Part model, mm, in its own coordinate system. Coordinates: 2 decimals unless noted, no trailing zeros. Loops run counter-clockwise (first coordinate to the right, second up) from the corner with the lowest first, then second, coordinate; pieces in that order, holes last. Notation, with made-up numbers: (-32, 83.25) -> (-27, 83.25) arc R34 ccw to (-27, 120.25) -> close; hole circle Ø3 at (-27, -36.75). An arc over 180 degrees is marked (long way). One line per item, written item: value. Start each with the question number.
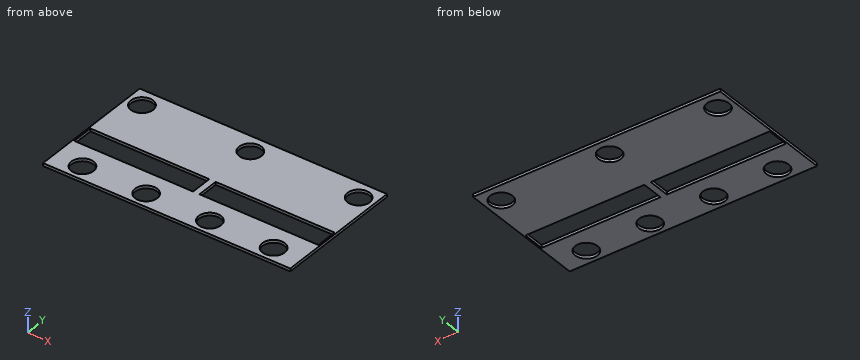
from build123d import *

# Parameters (mm, degrees)
SKETCH14_W                        = 80
SKETCH14_H                        = 42
SKETCH14_W_2                      = 3.75
SKETCH14_H_2                      = 3.75
BASE_WITH_CUTOUTS_DEPTH           = 3
SKETCH15_W                        = 4.3
SKETCH15_H                        = 4.8
SIPM_CUTOUTS_DEPTH                = 48.265209192
PADDLE_SUPPORT_TAPERS_DEPTH       = 2
SKETCH17_W                        = 80
SKETCH17_H                        = 25
PADDLE_SUPPORT_TOP_DEPTH          = 1
PADDLE_START                      = -4
SKETCH17_2_W                      = 80
SKETCH17_2_H                      = 25
PADDLE_SUPPORT_BOTTOM_DEPTH       = 1
PADDLE_SUPPORT_TAPER_TOP_SIZE     = 0.8
PADDLE_SUPPORT_TAPER_TOP_SIZE2    = 2.4
PADDLE_SUPPORT_TAPER_BOTTOM_SIZE  = 2.4
PADDLE_SUPPORT_TAPER_BOTTOM_SIZE2 = 0.8
SKETCH18_W                        = 4
SKETCH18_H                        = 22
SKETCH18_H_2                      = 14
BASE_THICKNESS_EXPANSION_DEPTH    = 80
BAFFLE_BASE_DEPTH                 = 2
BAFFLE_LIP_DEPTH                  = 2
BAFFLE_CHAMFER_1_2_SIZE           = 1.2
BAFFLE_CHAMFER_0_4_SIZE           = 0.4
INSERT_HOLES_PCB_D                = 3.3
INSERT_HOLES_PCB_DEPTH            = 4.2
INSERT_HOLES_PCB_CBORE_D          = 7
INSERT_HOLES_PCB_CBORE_DEPTH      = 1.4
JOINT_MOD_REACH                   = 56.854
SKETCH29_W                        = 37.3
SKETCH29_H                        = 6.8
CUT_EXTRUDE1_DEPTH                = 1.45
CHAMFER1_SIZE                     = 2
CHAMFER1_SIZE2                    = 5.494954839
SKETCH34_W                        = 81.499638764
SKETCH34_H                        = 0.25
CUT_EXTRUDE2_DEPTH                = 24
M1_6_CLEARANCE_HOLE1_D            = 1.8
SKETCH38_W                        = 104.100396554
SKETCH38_H                        = 54.802140704
CUT_EXTRUDE3_DEPTH                = 55.128573785
CUT_EXTRUDE4_DEPTH                = 0.05
SKETCH40_W                        = 1.2
SKETCH40_H                        = 9
CUT_EXTRUDE5_DEPTH                = 48.190677045
SKETCH41_W                        = 77.6
SKETCH41_H                        = 40.8
CUT_EXTRUDE6_DEPTH                = 0.5


with BuildPart() as part:
    # Sketch14 → BASE WITH CUTOUTS (new body)
    with BuildSketch(Plane.XY):
        with Locations((0, 4)):
            Rectangle(SKETCH14_W, SKETCH14_H)
        with Locations((10.45, 0)):
            Rectangle(SKETCH14_W_2, SKETCH14_H_2, mode=Mode.SUBTRACT)
        with Locations((4.15, 0)):
            Rectangle(SKETCH14_W_2, SKETCH14_H_2, mode=Mode.SUBTRACT)
        with Locations((16.75, 0)):
            Rectangle(SKETCH14_W_2, SKETCH14_H_2, mode=Mode.SUBTRACT)
        with Locations((23.05, 0)):
            Rectangle(SKETCH14_W_2, SKETCH14_H_2, mode=Mode.SUBTRACT)
        with Locations((29.35, 0)):
            Rectangle(SKETCH14_W_2, SKETCH14_H_2, mode=Mode.SUBTRACT)
        with Locations((35.65, 0)):
            Rectangle(SKETCH14_W_2, SKETCH14_H_2, mode=Mode.SUBTRACT)
        with Locations((-35.65, 0)):
            Rectangle(SKETCH14_W_2, SKETCH14_H_2, mode=Mode.SUBTRACT)
        with Locations((-29.35, 0)):
            Rectangle(SKETCH14_W_2, SKETCH14_H_2, mode=Mode.SUBTRACT)
        with Locations((-23.05, 0)):
            Rectangle(SKETCH14_W_2, SKETCH14_H_2, mode=Mode.SUBTRACT)
        with Locations((-16.75, 0)):
            Rectangle(SKETCH14_W_2, SKETCH14_H_2, mode=Mode.SUBTRACT)
        with Locations((-10.45, 0)):
            Rectangle(SKETCH14_W_2, SKETCH14_H_2, mode=Mode.SUBTRACT)
        with Locations((-4.15, 0)):
            Rectangle(SKETCH14_W_2, SKETCH14_H_2, mode=Mode.SUBTRACT)
    extrude(amount=-BASE_WITH_CUTOUTS_DEPTH)

    # Sketch15 → SIPM CUTOUTS (cut, through all)
    with BuildSketch(Plane(origin=(0, 0, -3), x_dir=(-1, 0, 0), z_dir=(0, 0, -1))):
        with Locations((-35.65, 0.125)):
            Rectangle(SKETCH15_W, SKETCH15_H)
        with Locations((-29.35, 0.125)):
            Rectangle(SKETCH15_W, SKETCH15_H)
        with Locations((-23.05, 0.125)):
            Rectangle(SKETCH15_W, SKETCH15_H)
        with Locations((-16.75, 0.125)):
            Rectangle(SKETCH15_W, SKETCH15_H)
        with Locations((-10.45, 0.125)):
            Rectangle(SKETCH15_W, SKETCH15_H)
        with Locations((-4.15, 0.125)):
            Rectangle(SKETCH15_W, SKETCH15_H)
        with Locations((4.15, 0.125)):
            Rectangle(SKETCH15_W, SKETCH15_H)
        with Locations((10.45, 0.125)):
            Rectangle(SKETCH15_W, SKETCH15_H)
        with Locations((16.75, 0.125)):
            Rectangle(SKETCH15_W, SKETCH15_H)
        with Locations((23.05, 0.125)):
            Rectangle(SKETCH15_W, SKETCH15_H)
        with Locations((29.35, 0.125)):
            Rectangle(SKETCH15_W, SKETCH15_H)
        with Locations((35.65, 0.125)):
            Rectangle(SKETCH15_W, SKETCH15_H)
    extrude(amount=-SIPM_CUTOUTS_DEPTH, mode=Mode.SUBTRACT)

    # Sketch16 → PADDLE SUPPORT - TAPERS (add, symmetric)
    with BuildSketch(Plane(origin=(0, 0, 0), x_dir=(1, 0, 0), z_dir=(0, 1, 0))):
        Polygon((40, 0), (37.691381155, 0), (40, -16.789955233), align=None)
        Polygon((0, 0), (2.308618845, 0), (0, -16.789955233), (-2.308618845, 0), align=None)
        Polygon((-40, -16.789955233), (-37.691381155, 0), (-40, 0), align=None)
    extrude(amount=PADDLE_SUPPORT_TAPERS_DEPTH, both=True)

    # Sketch17 → PADDLE SUPPORT - TOP (add)
    with BuildSketch(Plane(origin=(0, 2, 0), x_dir=(1, 0, 0), z_dir=(0, 1, 0))):
        with Locations((0, -12.5)):
            Rectangle(SKETCH17_W, SKETCH17_H)
    extrude(amount=PADDLE_SUPPORT_TOP_DEPTH)

    # Sketch17<2> → PADDLE SUPPORT - BOTTOM (add)
    with BuildSketch(Plane(origin=(0, 2, 0), x_dir=(1, 0, 0), z_dir=(0, 1, 0)).offset(PADDLE_START)):
        with Locations((0, -12.5)):
            Rectangle(SKETCH17_2_W, SKETCH17_2_H)
    extrude(amount=-PADDLE_SUPPORT_BOTTOM_DEPTH)

    # PADDLE SUPPORT - TAPER TOP
    paddle_support_taper_top_edges = [part.edges().sort_by_distance(p)[0] for p in [
        (0, 3, 25),
    ]]
    paddle_support_taper_top_side = [part.faces().sort_by_distance(p)[0] for p in [
        (0, 2.5, 25),
    ]]
    chamfer(paddle_support_taper_top_edges, length=PADDLE_SUPPORT_TAPER_TOP_SIZE, length2=PADDLE_SUPPORT_TAPER_TOP_SIZE2, reference=paddle_support_taper_top_side[0])

    # PADDLE SUPPORT - TAPER BOTTOM
    paddle_support_taper_bottom_edges = [part.edges().sort_by_distance(p)[0] for p in [
        (0, -3, 25),
    ]]
    paddle_support_taper_bottom_side = [part.faces().sort_by_distance(p)[0] for p in [
        (0, -3, 12.5),
    ]]
    chamfer(paddle_support_taper_bottom_edges, length=PADDLE_SUPPORT_TAPER_BOTTOM_SIZE, length2=PADDLE_SUPPORT_TAPER_BOTTOM_SIZE2, reference=paddle_support_taper_bottom_side[0])

    # Sketch18 → BASE - THICKNESS EXPANSION (add)
    with BuildSketch(Plane(origin=(40, 0, 0), x_dir=(0, 0, -1), z_dir=(1, 0, 0))):
        with Locations((-2, 14)):
            Rectangle(SKETCH18_W, SKETCH18_H)
        with Locations((-2, -10)):
            Rectangle(SKETCH18_W, SKETCH18_H_2)
    extrude(amount=-BASE_THICKNESS_EXPANSION_DEPTH)

    # Sketch19 → BAFFLE - BASE (cut)
    with BuildSketch(Plane(origin=(0, 0, -3), x_dir=(-1, 0, 0), z_dir=(0, 0, -1))):
        Polygon((-40, 16), (-39.2, 16), (-39.2, -16.2), (39.2, -16.2), (39.2, 16), (40, 16), (40, -17), (-40, -17), align=None)
    extrude(amount=-BAFFLE_BASE_DEPTH, mode=Mode.SUBTRACT)

    # Sketch20 → BAFFLE - LIP (cut)
    with BuildSketch(Plane(origin=(0, 0, -1), x_dir=(-1, 0, 0), z_dir=(0, 0, -1))):
        Polygon((-40, 16), (-40, -17), (40, -17), (40, 16), (38.8, 16), (38.8, -15.8), (-38.8, -15.8), (-38.8, 16), align=None)
    extrude(amount=-BAFFLE_LIP_DEPTH, mode=Mode.SUBTRACT)

    # BAFFLE - CHAMFER 1.2
    baffle_chamfer_1_2_edges = [part.edges().sort_by_distance(p)[0] for p in [
        (-40, -0.5, 1),
        (0, -17, 1),
        (40, -0.5, 1),
    ]]
    chamfer(baffle_chamfer_1_2_edges, length=BAFFLE_CHAMFER_1_2_SIZE - 0.0001)  # a hair under: the kernel refuses the full size

    # BAFFLE - CHAMFER 0.4
    baffle_chamfer_0_4_edges = [part.edges().sort_by_distance(p)[0] for p in [
        (39.2, -0.1, -1),
        (-39.2, -0.1, -1),
        (0, -16.2, -1),
    ]]
    chamfer(baffle_chamfer_0_4_edges, length=BAFFLE_CHAMFER_0_4_SIZE - 0.0001)  # a hair under: the kernel refuses the full size

    # INSERT HOLES - PCB
    with Locations(Plane(origin=(0, 0, -3), x_dir=(-1, 0, 0), z_dir=(0, 0, -1))):
        with Locations((-30, -11), (-10, -11), (10, -11), (30, -11), (-34, 19.5), (0, 19.5), (34, 19.5)):
            CounterBoreHole(INSERT_HOLES_PCB_D / 2, INSERT_HOLES_PCB_CBORE_D / 2, INSERT_HOLES_PCB_CBORE_DEPTH, depth=INSERT_HOLES_PCB_DEPTH)

    # Sketch26 → JOINT MOD (cut, up to next)
    with BuildSketch(Plane(origin=(0, 0, -3), x_dir=(-1, 0, 0), z_dir=(0, 0, -1)), mode=Mode.PRIVATE) as joint_mod_sk1:
        Polygon((-38.8, 16), (-38.8, -15.8), (38.8, -15.8), (38.8, 16), (39.2, 16), (39.2, -16.2), (-39.2, -16.2), (-39.2, 16), align=None)
    joint_mod_tool1 = extrude(joint_mod_sk1.sketch, amount=-JOINT_MOD_REACH, mode=Mode.PRIVATE) & part.part
    add(joint_mod_tool1.solids().sort_by_distance((38.884755, 0.1, -3))[0], mode=Mode.SUBTRACT)

    # Sketch29 → Cut-Extrude1 (cut)
    with BuildSketch(Plane(origin=(0, 0, -3), x_dir=(-1, 0, 0), z_dir=(0, 0, -1))):
        with Locations((-19.65, 0.125)):
            Rectangle(SKETCH29_W, SKETCH29_H)
        with Locations((19.65, 0.125)):
            Rectangle(SKETCH29_W, SKETCH29_H)
    extrude(amount=-CUT_EXTRUDE1_DEPTH, mode=Mode.SUBTRACT)

    # Chamfer1
    chamfer1_edges = [part.edges().sort_by_distance(p)[0] for p in [
        (0, 3, 4),
    ]]
    chamfer1_side = [part.faces().sort_by_distance(p)[0] for p in [
        (0, 3, 13.3),
    ]]
    chamfer(chamfer1_edges, length=CHAMFER1_SIZE, length2=CHAMFER1_SIZE2, reference=chamfer1_side[0])

    # Sketch34 → Cut-Extrude2 (cut)
    with BuildSketch(Plane.XY.offset(25)):
        Rectangle(SKETCH34_W, SKETCH34_H)
    extrude(amount=-CUT_EXTRUDE2_DEPTH, mode=Mode.SUBTRACT)

    # M1.6 Clearance Hole1 (through all)
    with Locations(Plane(origin=(0, -3, 0), x_dir=(-1, 0, 0), z_dir=(0, -1, 0))):
        with Locations((0, -8)):
            Hole(M1_6_CLEARANCE_HOLE1_D / 2)

    # Sketch38 → Cut-Extrude3 (cut, through all)
    with BuildSketch(Plane(origin=(0, 0, -1.55), x_dir=(-1, 0, 0), z_dir=(0, 0, -1))):
        Rectangle(SKETCH38_W, SKETCH38_H)
    extrude(amount=-CUT_EXTRUDE3_DEPTH, mode=Mode.SUBTRACT)

    # Sketch39 → Cut-Extrude4 (cut)
    with BuildSketch(Plane.XY.offset(-1.55)):
        Polygon((40, 25), (-40, 25), (-40, 16), (-38.8, 16), (-38.8, -15.8), (38.8, -15.8), (38.8, 16), (40, 16), align=None)
    extrude(amount=-CUT_EXTRUDE4_DEPTH, mode=Mode.SUBTRACT)

    # Sketch40 → Cut-Extrude5 (cut, through all)
    with BuildSketch(Plane.XY.offset(-1.6)):
        with Locations((-39.4, 20.5)):
            Rectangle(SKETCH40_W, SKETCH40_H)
        with Locations((39.4, 20.5)):
            Rectangle(SKETCH40_W, SKETCH40_H)
    extrude(amount=-CUT_EXTRUDE5_DEPTH, mode=Mode.SUBTRACT)

    # Sketch41 → Cut-Extrude6 (cut)
    with BuildSketch(Plane.XY.offset(-1.6)):
        with Locations((0, 4.6)):
            Rectangle(SKETCH41_W, SKETCH41_H)
    extrude(amount=-CUT_EXTRUDE6_DEPTH, mode=Mode.SUBTRACT)


solid = part.part
1) Pin check, flat tip, straight feed: pin 1 Ø11 at (x, y) = (-34, 19.5) entering from -Z. Stop position of the tip, or through.
2) Probe line 1 (Y direction, x = 34, z = -2.65) (3 decimals); line 2 (Y direction, x = 0, z = -2.5); line 3 (Y direction, x = -20, z = -2.65) (3 decimals). List the from-to ranges inside material, lowest first. Write a range as from..to.
3) Slice it at A-A (x = 0). Give the cut face in (y, z), then the cut area to 3 significant figures.
4) Slice it at D-D (x = 10). Give the cut face in (y, z) (3 decimals).
5) Slice it at C-C (y = -2). Give the cut face in (x, z).
6) Slice it at B-B (z = -2.25). State how many separate pieces and enclosed holes the cut face has, then the cut area to 3 significant figures.
Check sheet entries:
1. pin 1: stops at z = -3
2. line 1: y = -15.8..-3.275, 3.525..16, 23..25
2. line 2: y = -15.8..16, 23..25
2. line 3: y = -15.8..-3.275, 3.525..25
3. outline: (-15.8, -3) -> (16, -3) -> (16, -2.1) -> (-15.8, -2.1) -> close; (23, -3) -> (25, -3) -> (25, -2.1) -> (23, -2.1) -> close
3. area: 30.4 mm^2
4. outline: (-15.8, -3) -> (-14.5, -3) -> (-14.5, -2.1) -> (-15.8, -2.1) -> close; (-7.5, -3) -> (-3.275, -3) -> (-3.275, -2.1) -> (-7.5, -2.1) -> close; (3.525, -3) -> (25, -3) -> (25, -2.1) -> (3.525, -2.1) -> close
5. outline: (-38.8, -3) -> (-38.3, -3) -> (-38.3, -2.1) -> (-38.8, -2.1) -> close; (-1, -3) -> (1, -3) -> (1, -2.1) -> (-1, -2.1) -> close; (38.3, -3) -> (38.8, -3) -> (38.8, -2.1) -> (38.3, -2.1) -> close
6. separate pieces: 1
6. enclosed holes: 9
6. area: 2,390 mm^2
